Geometry check sheet. Reference: the model listing, model coordinates, mm. A direction names the side the tool comes from. Round coordinates to 2 decimals unless told otherwise and drop trailing zeros. Write each loop counter-clockwise with the first axis right and the second up, starting at its lowest first coordinate (ties: lowest second). Pieces come first, ordered by that corner, then holes. Notation, with made-up numbers: M 84,73 L 110,73 A23 ccw 110,110 Z; hole C -34.75,3 d5. An arc over 180 degrees is marked long. Answer in a Markdown table with one row per item. Add a question column.
from build123d import *

# Parameters (mm, degrees)
F1_DEPTH        = 70
F2_W            = 28.213582236
F2_H            = 30.1489157287
F3_DEPTH        = 52
F4_R            = 5
F6_DEPTH        = 18
F7_W            = 4
F7_H            = 4
F8_DEPTH        = 70.001
F9_R            = 4
F10_DEPTH       = 40.001
F11_R           = 9
F12_DEPTH       = 6
F14_D           = 4
F14_DEPTH       = 5.5
F14_TIP         = 1.2017212381
F17_D           = 3.2
F17_DEPTH       = 8
F17_CBORE_D     = 6.5
F17_CBORE_DEPTH = 3
F17_TIP         = 0.9613769904
F18_D           = 3.2
F18_DEPTH       = 8
F18_TIP         = 0.9613769904
F19_D           = 4.3
F19_DEPTH       = 8
F19_TIP         = 1.2918503309


with BuildPart() as f1:
    # F0 (on Front) → F1 (new body)
    with BuildSketch(Plane.XZ):
        Polygon((28.2647607103, 22.518672328), (-31.7352392897, 22.518672328), (-31.7352392897, -17.481327672), (4.2647607103, -17.481327672), (4.2647607103, -9.1914124787), (4.2647607103, 3.018672328), (13.7647607103, 12.518672328), (23.2647607103, 3.018672328), (28.2647607103, 3.018672328), align=None)
    extrude(amount=F1_DEPTH)

    # F2 (on face) → F3 (cut)
    with BuildSketch(Plane(origin=(0, 0, 0), x_dir=(-1, 0, 0), z_dir=(0, 1, 0))):
        with Locations((25.8420304077, 12.5931301923)):
            Rectangle(F2_W, F2_H)
    extrude(amount=-F3_DEPTH, mode=Mode.SUBTRACT)

    # F4
    f4_edges = [f1.edges().sort_by_distance(p)[0] for p in [
        (-31.735239, -61, 22.518672),
        (-31.735239, -35, -17.481328),
    ]]
    fillet(f4_edges, radius=F4_R)

    # F5 (on face) → F6 (cut, through all)
    with BuildSketch(Plane.XZ.offset(70)):
        with BuildLine():
            Line((-20.0560601684, 1.518672328), (-20.0560601684, 7.3947146633))
            ThreePointArc((-20.0560601684, 7.3947146633), (-21.9196415591, 19.8659942674), (-23.0560601684, 7.3075587236))
            Line((-23.0560601684, 7.3075587236), (-23.0560601684, 1.518672328))
            ThreePointArc((-23.0560601684, 1.518672328), (-21.5560601684, 0.018672328), (-20.0560601684, 1.518672328))
        make_face()
    extrude(amount=-F6_DEPTH, mode=Mode.SUBTRACT)

    # F7 (on face) → F8 (cut, through all)
    with BuildSketch(Plane.XZ.offset(70)):
        with Locations((13.7647607103, 12.518672328)):
            Rectangle(F7_W, F7_H)
    extrude(amount=-F8_DEPTH, mode=Mode.SUBTRACT)

    # F9 (on face) → F10 (cut, through all)
    with BuildSketch(Plane(origin=(0, 0, -17.481327672), x_dir=(1, 0, 0), z_dir=(0, 0, -1))):
        with Locations((-1.7352392897, 35)):
            Circle(F9_R)
    extrude(amount=-F10_DEPTH, mode=Mode.SUBTRACT)

    # F11 (on face) → F12 (cut)
    with BuildSketch(Plane.XY.offset(22.518672328)):
        with Locations((-1.7352392897, -35)):
            Circle(F11_R)
    extrude(amount=-F12_DEPTH, mode=Mode.SUBTRACT)

    # F14
    with Locations(Plane(origin=(0, 0, -17.481327672), x_dir=(1, 0, 0), z_dir=(0, 0, -1))):
        with Locations((-19.7227925898, 50), (-20.3082847504, 20)):
            Hole(F14_D / 2, depth=F14_DEPTH)
            with Locations((0, 0, -(F14_DEPTH + F14_TIP / 2))):  # 118° drill point
                Cone(0, F14_D / 2, F14_TIP, mode=Mode.SUBTRACT)

    # F17
    with Locations(Plane(origin=(-31.7352392897, 0, 0), x_dir=(0, -1, 0), z_dir=(-1, 0, 0))):
        with Locations((61, 4.518672328)):
            CounterBoreHole(F17_D / 2, F17_CBORE_D / 2, F17_CBORE_DEPTH, depth=F17_DEPTH)
            with Locations((0, 0, -(F17_DEPTH + F17_TIP / 2))):  # 118° drill point
                Cone(0, F17_D / 2, F17_TIP, mode=Mode.SUBTRACT)

    # F18 (one way)
    with BuildSketch(Plane(origin=(-20.0560601684, 0, 0), x_dir=(0, -1, 0), z_dir=(-1, 0, 0))):
        with Locations((61, 4.518672328)):
            Circle(F18_D / 2)
    extrude(amount=-F18_DEPTH, mode=Mode.SUBTRACT)
    with Locations(Plane(origin=(-20.0560601684, 0, 0), x_dir=(0, -1, 0), z_dir=(-1, 0, 0))):
        with Locations((61, 4.518672328)):
            with Locations((0, 0, -(F18_DEPTH + F18_TIP / 2))):  # 118° drill point
                Cone(0, F18_D / 2, F18_TIP, mode=Mode.SUBTRACT)

    # F19
    with Locations(Plane(origin=(-31.7352392897, 0, 0), x_dir=(0, -1, 0), z_dir=(-1, 0, 0))):
        with Locations((62, 13.518672328)):
            Hole(F19_D / 2, depth=F19_DEPTH)
            with Locations((0, 0, -(F19_DEPTH + F19_TIP / 2))):  # 118° drill point
                Cone(0, F19_D / 2, F19_TIP, mode=Mode.SUBTRACT)


solid = f1.part
Item 1: Access from +Z, -Z, +X, -X, +Y, -Y to the whole of each face (thin tool, end or side, straight path). Record for faces 1 (the cylindrical face through (-29.694, -59.949, 14.164)), 2 (the cylindrical face through (-2.907, -26.077, 19.561)), 3 (the cylindrical face through (-20.048, -21.983, -14.693)), 4 (the flat face through (14, -35, 14.519)), 5 (the flat face through (-11.735, -26, 10)).
Item 2: Section check D-D, the plane y = -46. Record the boundary of the cut face in (x, z).
Item 3: Section check B-B, the plane y = -35. Record the boundary of the cut face in (x, z).
Item 4: Section check A-A, the plane z = 19. Record the boundary of the cut face in (x, y).
Item 5: Section check C-C, the plane z = 9. Record the boundary of the cut face in (x, y), and give its area (3 significant figures).
Item 6: Gauge pin test, flat ends, axial feed: pin 1 Ø4 at (y, z) = (-21, 11.5) entering from -X; pin 2 Ø10 at (x, y) = (-20, -15.5) entering from +Z; pin 3 Ø4 at (y, z) = (-61, 4.52) entering from -X; pin 4 Ø7 at (x, y) = (-1.74, -35) entering from -Z. Record the tip position at first contact, or that the pin passes through.
Item 7: Scan lines: probe 1 along X at (y, z) = (-26, 12); probe 2 along Y at (x, z) = (-1.5, 0); probe 3 along X at (y, z) = (-35, -3). Record each from-to range of solid material in increasing order. Write a range as from..to.
Item 8: Mould release check, pull along Y, two halves, no side actions. Record for faces 6 (the cylindrical face through (-19.289, -48.048, -14.693)), 7 (the flat face through (-23.056, -61, 3)), 8 (the flat face through (-2, 0, 3)): +Y half, -Y half, draft (parallel to the pull), parting line (faces both ways), or undercut.
Result sheet:
| question | item | result |
|---|---|---|
| 1 | face 1 | -X |
| 1 | face 2 | +Z |
| 1 | face 3 | -Z |
| 1 | face 4 | -Z, +Y, -Y |
| 1 | face 5 | +Z, -X, +Y |
| 2 | outline | M -31.74,-12.48 A5 ccw -26.74,-17.48 L 4.26,-17.48 L 4.26,3.02 L 11.76,10.52 L 11.76,14.52 L 15.76,14.52 L 15.76,10.52 L 23.26,3.02 L 28.26,3.02 L 28.26,22.52 L -11.74,22.52 L -11.74,-2.48 L -31.74,-2.48 Z |
| 3 | outline | M -31.74,-12.48 A5 ccw -26.74,-17.48 L -5.74,-17.48 L -5.74,16.52 L -10.74,16.52 L -10.74,22.52 L -11.74,22.52 L -11.74,-2.48 L -31.74,-2.48 Z; M 2.26,-17.48 L 4.26,-17.48 L 4.26,3.02 L 11.76,10.52 L 11.76,14.52 L 15.76,14.52 L 15.76,10.52 L 23.26,3.02 L 28.26,3.02 L 28.26,22.52 L 7.26,22.52 L 7.26,16.52 L 2.26,16.52 Z |
| 4 | outline | M -31.51,-70 L -24.94,-70 L -24.94,-52 L -31.51,-52 Z; M -18.53,-70 L 28.26,-70 L 28.26,0 L -11.74,0 L -11.74,-52 L -18.53,-52 Z; hole C -1.74,-35 d18 |
| 5 | outline | M -31.74,-70 L -26.2,-70 L -26.2,-52 L -31.74,-52 Z; M -17.27,-70 L 10.25,-70 L 10.25,0 L -11.74,0 L -11.74,-52 L -17.27,-52 Z; M 17.28,-70 L 28.26,-70 L 28.26,0 L 17.28,0 Z; hole C -1.74,-35 d8 |
| 5 | area | 2,460 mm^2 |
| 6 | pin 1 | stops at x = -11.74 |
| 6 | pin 2 | stops at z = -2.48 |
| 6 | pin 3 | stops at x = -28.74 |
| 6 | pin 4 | passes through |
| 7 | probe 1 | x = -11.74..11.76, 15.76..28.26 |
| 7 | probe 2 | y = -70..-38.99, -31.01..0 |
| 7 | probe 3 | x = -31.74..-5.74, 2.26..4.26 |
| 8 | face 6 | undercut |
| 8 | face 7 | draft |
| 8 | face 8 | +Y half |
